Geometry check sheet. Reference: the model listing, model coordinates, mm. Face numbers are marked on the shaded views. A direction names the side the tool comes from. Coordinates: 2 decimals unless noted, no trailing zeros. Loops run counter-clockwise (first coordinate to the right, second up) from the corner with the lowest first, then second, coordinate; pieces in that order, holes last.
from build123d import *

# Parameters (mm, degrees)
BOSS_EXTRUDE1_DEPTH = 88.9
SKETCH2_R           = 3.175
CUT_EXTRUDE1_DEPTH  = 76.2
SKETCH3_R           = 4.7625
CUT_EXTRUDE2_DEPTH  = 39.1


with BuildPart() as part:
    # Sketch1 → Boss-Extrude1 (new body)
    with BuildSketch(Plane.XY):
        Polygon((0, 0), (0, 38.1), (6.35, 38.1), (6.35, 6.35), (38.1, 6.35), (38.1, 0), align=None)
    extrude(amount=BOSS_EXTRUDE1_DEPTH)

    # Sketch2 → Cut-Extrude1 (cut)
    with BuildSketch(Plane.ZY):
        with Locations((12.95, 28.575)):
            Circle(SKETCH2_R)
        with Locations((75.95, 28.575)):
            Circle(SKETCH2_R)
        with BuildLine():
            ThreePointArc((18.104961724, 38.1), (44.45, 16.733289595), (70.795038276, 38.1))
            Line((70.795038276, 38.1), (18.104961724, 38.1))
        make_face()
    extrude(amount=-CUT_EXTRUDE1_DEPTH, mode=Mode.SUBTRACT)

    # Sketch3 → Cut-Extrude2 (cut, through all)
    with BuildSketch(Plane.XZ):
        with Locations((25.4, 69.85)):
            Circle(SKETCH3_R)
        with Locations((25.4, 19.05)):
            Circle(SKETCH3_R)
    extrude(amount=-CUT_EXTRUDE2_DEPTH, mode=Mode.SUBTRACT)


solid = part.part
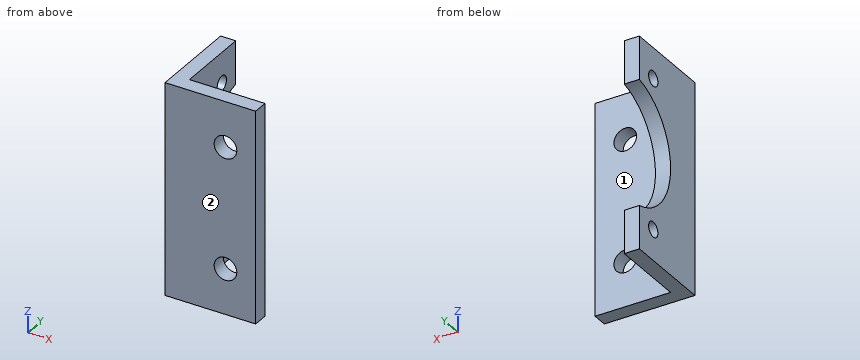
1) Section check A-A on x = 25.4. Record the cut outline in (y, z), and give its area (3 significant figures).
Data:
outline: (0, 0) - (6.35, 0) - (6.35, 14.29) - (0, 14.29) - close; (0, 23.81) - (6.35, 23.81) - (6.35, 65.09) - (0, 65.09) - close; (0, 74.61) - (6.35, 74.61) - (6.35, 88.9) - (0, 88.9) - close
area: 444 mm2
2) Section check B-B on z = 12.95. Record the cut outline in (x, y), and give its area (3 significant figures).
Data:
outline: (0, 0) - (38.1, 0) - (38.1, 6.35) - (6.35, 6.35) - (6.35, 25.4) - (0, 25.4) - close; (0, 31.75) - (6.35, 31.75) - (6.35, 38.1) - (0, 38.1) - close
area: 403 mm2
3) Section check D-D on z = 82. Record the cut outline in (x, y), and give its area (3 significant figures).
Data:
outline: (0, 0) - (38.1, 0) - (38.1, 6.35) - (6.35, 6.35) - (6.35, 38.1) - (0, 38.1) - close
area: 444 mm2
4) Section check C-C on y = 33. Record the cut outline in (x, z).
Data:
outline: (0, 0) - (6.35, 0) - (6.35, 19.72) - (0, 19.72) - close; (0, 69.18) - (6.35, 69.18) - (6.35, 88.9) - (0, 88.9) - close
5) Access from +Z, -Z, +X, -X, +Y, -Y to the whole of each face (thin tool, end or side, straight path). Record for the marked faces 1 and 2.
Data:
face 1: +Z, -Z, +X, +Y
face 2: +Z, -Z, +X, -X, -Y
6) Material ranges on probe 1 along Z at (x, y) = (25.4, 4); probe 2 along X at (y, z) = (9, 72), recorded low to high.
Data:
probe 1: z = 0 to 14.29, 23.81 to 65.09, 74.61 to 88.9
probe 2: x = 0 to 6.35
7) Depth check by flat-ended pin: pin 1 (8.5 mm diameter, centred on x = 25.4, z = 69.85, fed in from +Y); pin 2 (7.5 mm diameter, centred on y = 28.575, z = 12.95, fed in from +X); pin 3 (1 mm diameter, centred on x = 22.5, z = 75, fed in from +Y). Enter the tip coordinate at first touch or a pass-through.
Data:
pin 1: passes through
pin 2: stops at x = 6.35
pin 3: stops at y = 6.35
